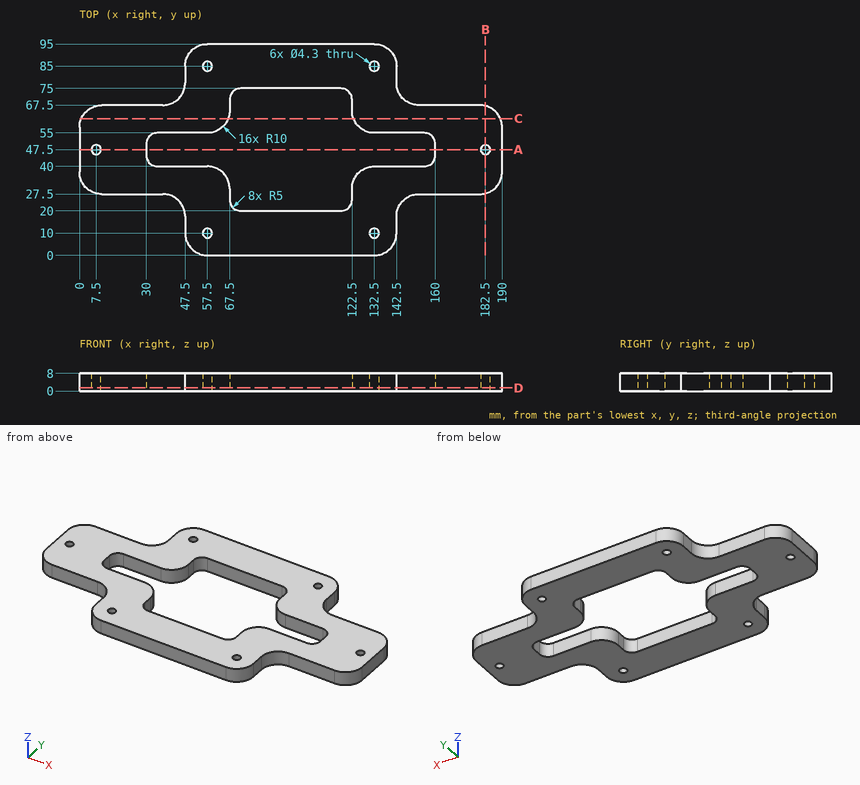
Print and shaded views of the part. All mm, measured from the part's lowest x, y and z. Give positions to 0.01 mm unless a question says otherwise; leave off trailing zeros. Write each loop counter-clockwise with the first axis right and the second up, starting at its lowest first coordinate (ties: lowest second). Pieces come first, ordered by that corner, then holes. Notation, with made-up numbers: (69, -1.5) -> (88, -1.5) arc R25 cw to (88, 15.5) -> close; hole circle Ø8 at (36, 30.5). An arc over 180 degrees is marked (long way). Write item = value, one per line.
(1) Slice it at D-D, the plane z = 1.5. Give the number of separate pieces and of enclosed holes in the cut face, then the cut area to 3 significant figures.
Determined:
separate_pieces = 1
enclosed_holes = 7
area = 8,460 mm2
(2) Slice it at C-C, the plane y = 61.5. Give the cut face in (x, z).
Determined:
outline = (0.83, 0) -> (66.87, 0) -> (66.87, 8) -> (0.83, 8) -> close; (123.13, 0) -> (189.17, 0) -> (189.17, 8) -> (123.13, 8) -> close
(3) Slice it at B-B, the plane x = 182.5. Give the cut face in (y, z).
Determined:
outline = (27.82, 0) -> (45.35, 0) -> (45.35, 8) -> (27.82, 8) -> close; (49.65, 0) -> (67.18, 0) -> (67.18, 8) -> (49.65, 8) -> close
(4) Flat gauge pins, fed straight in: P1, Ø2.5, axis at x = 26.5, z = 2.5, coming from the +Y side; P2, Ø4, axis at x = 27, z = 5.5, coming from the -Y side; P3, Ø4, axis at y = 35, z = 1, coming from the -X side. Where does each tip first touch, or does it go through?
Determined:
P1 = 67.5
P2 = 27.5
P3 = 0.01
(5) Probe line 1 along Y through (x, z) = (57.5, 4); line 2 along Y through (x, z) = (83, 6.5); line 3 along X through (y, z) = (83.5, 6). List the from-to ranges inside material, lowest first.
Determined:
line_1 = 0 to 7.85, 12.15 to 40, 55 to 82.85, 87.15 to 95
line_2 = 0 to 20, 75 to 95
line_3 = 47.5 to 55.96, 59.04 to 130.96, 134.04 to 142.5
(6) Slice it at A-A, the plane y = 47.5. Give the cut face in (x, z).
Determined:
outline = (0, 0) -> (5.35, 0) -> (5.35, 8) -> (0, 8) -> close; (9.65, 0) -> (30, 0) -> (30, 8) -> (9.65, 8) -> close; (160, 0) -> (180.35, 0) -> (180.35, 8) -> (160, 8) -> close; (184.65, 0) -> (190, 0) -> (190, 8) -> (184.65, 8) -> close
